Can you work these out from the model? Positions are in its coordinate system, mm. Face numbers are marked on the shaded views. A direction names the side the tool comes from. Coordinates: 2 decimals unless noted, no trailing zeros. Order: outer loops, then holes, each group sorted by start corner. A loop starts at its lowest first (then second) coordinate and runs counter-clockwise, first axis right, second up. Notation, with made-up numbers: (62.5, 70) -> (91.5, 70) arc R33 ccw to (91.5, 99) -> close; hole circle Ø9 at (51.25, -39). An arc over 180 degrees is marked (long way). Write item = value, one per line.
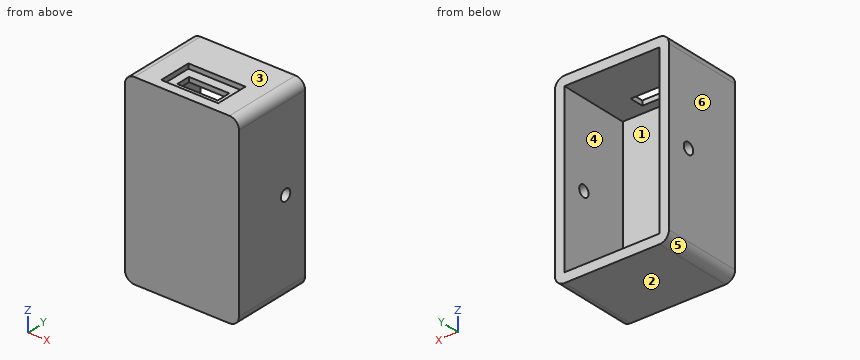
```python
from build123d import *

# Parameters (mm, degrees)
IZIM1_W                     = 24
IZIM1_H                     = 39
Y_KSEKLIK_EKSTR_ZYON1_DEPTH = 17
RADYUS1_R                   = 2
BO_ALTMA1_START             = -12.470588235
BO_ALTMA1_OUTLINE_W         = 15
BO_ALTMA1_OUTLINE_H         = 35
BO_ALTMA1_DEPTH             = 20
IZIM2_W                     = 8.5
IZIM2_H                     = 3
KES_EKSTR_ZYON1_DEPTH       = 17
IZIM3_W                     = 12
IZIM3_H                     = 7
KES_EKSTR_ZYON2_DEPTH       = 1
IZIM5_R                     = 1.2
KES_EKSTR_ZYON3_DEPTH       = 30


# Read off the part's stored shape, not the designer's step: İç Boşaltma1
with BuildPart() as part:
    # Çizim1 → Yükseklik-Ekstrüzyon1 (new body)
    with BuildSketch(Plane(origin=(0, 0, 0), x_dir=(1, 0, 0), z_dir=(0, 1, 0))):
        with Locations((-2.470588235, -5.382352941)):
            Rectangle(IZIM1_W, IZIM1_H)
    extrude(amount=Y_KSEKLIK_EKSTR_ZYON1_DEPTH)

    # Radyus1
    radyus1_edges = [part.edges().sort_by_distance(p)[0] for p in [
        (-14.470588235, 8.5, -14.117647059),
        (9.529411765, 8.5, -14.117647059),
        (9.529411765, 8.5, 24.882352941),
        (-14.470588235, 8.5, 24.882352941),
    ]]
    fillet(radyus1_edges, radius=RADYUS1_R)

    # İç Boşaltma1 outline → İç Boşaltma1 (cut)
    with BuildSketch(Plane.YZ.offset(BO_ALTMA1_START)):
        with Locations((9.5, 5.382352941)):
            Rectangle(BO_ALTMA1_OUTLINE_W, BO_ALTMA1_OUTLINE_H)
    extrude(amount=BO_ALTMA1_DEPTH, mode=Mode.SUBTRACT)

    # Çizim2 → Kes-Ekstrüzyon1 (cut)
    with BuildSketch(Plane.XY.offset(24.882352941)):
        with Locations((-2.470588235, 5.5)):
            Rectangle(IZIM2_W, IZIM2_H)
    extrude(amount=-KES_EKSTR_ZYON1_DEPTH, mode=Mode.SUBTRACT)

    # Çizim3 → Kes-Ekstrüzyon2 (cut)
    with BuildSketch(Plane.XY.offset(24.882352941)):
        with Locations((-2.470588235, 5.5)):
            Rectangle(IZIM3_W, IZIM3_H)
    extrude(amount=-KES_EKSTR_ZYON2_DEPTH, mode=Mode.SUBTRACT)

    # Çizim5 → Kes-Ekstrüzyon3 (cut)
    with BuildSketch(Plane(origin=(9.529411765, 0, 0), x_dir=(0, 0, -1), z_dir=(1, 0, 0))):
        with Locations((-5.382352941, 12)):
            Circle(IZIM5_R)
    extrude(amount=-KES_EKSTR_ZYON3_DEPTH, mode=Mode.SUBTRACT)


solid = part.part
```
Item 1: For the marked faces 1 and 2, which set-ups out of +Z, -Z, +X, -X, +Y, -Y let a thin tool reach every point of the face, with its end or its side?
A:
face_1 = +Y
face_2 = -Z, +X, -X, +Y, -Y
Item 2: I want a section at D-D, the plane z = -3.5. Please give me the cut outline in (x, y).
A:
outline = (-14.47, 0) -> (9.53, 0) -> (9.53, 17) -> (7.53, 17) -> (7.53, 2) -> (-12.47, 2) -> (-12.47, 17) -> (-14.47, 17) -> close
Item 3: I want a section at C-C, the plane y = 14. Please give me the cut outline in (x, z), plus the area to 3 significant figures.
A:
outline = (-14.47, -12.12) arc R2 ccw to (-12.47, -14.12) -> (7.53, -14.12) arc R2 ccw to (9.53, -12.12) -> (9.53, 22.88) arc R2 ccw to (7.53, 24.88) -> (-12.47, 24.88) arc R2 ccw to (-14.47, 22.88) -> close; hole (-12.47, -12.12) -> (7.53, -12.12) -> (7.53, 22.88) -> (-12.47, 22.88) -> close
area = 233 mm2
Item 4: I'm going to push flat-ended pins straight in: P1, Ø2, axis at x = -0.5, y = 7.5, coming from the +Z side; P2, Ø0.8, axis at x = -1, z = 23.5, coming from the -Y side; P3, Ø1.1, axis at y = 5.5, z = 24, coming from the -X side; P4, Ø1.4, axis at y = 12, z = 5.38, coming from the +X side. Where does each tip first touch, or does it pass through?
A:
P1 = 23.88
P2 = 0
P3 = -14.39
P4 = through
Item 5: If we mould it in two halves opening along Z, with no side actions, what happens to the marked faces 3, 4, 5 and 6? For each: pulls with the +Z half, pulls with the -Z half, needs draft (parallel to the pull), parting line crosses it, or undercut.
A:
face_3 = pulls with the +Z half
face_4 = undercut
face_5 = pulls with the -Z half
face_6 = needs draft
Item 6: I want a section at B-B, the plane y = 12. Please give me the cut outline in (x, z).
A:
outline = (-14.47, -12.12) arc R2 ccw to (-12.47, -14.12) -> (7.53, -14.12) arc R2 ccw to (9.53, -12.12) -> (9.53, 4.18) -> (7.53, 4.18) -> (7.53, -12.12) -> (-12.47, -12.12) -> (-12.47, 4.18) -> (-14.47, 4.18) -> close; (-14.47, 6.58) -> (-12.47, 6.58) -> (-12.47, 22.88) -> (7.53, 22.88) -> (7.53, 6.58) -> (9.53, 6.58) -> (9.53, 22.88) arc R2 ccw to (7.53, 24.88) -> (-12.47, 24.88) arc R2 ccw to (-14.47, 22.88) -> close
Item 7: I want a section at A-A, the plane x = 0.75. Please give me the cut outline in (y, z).
A:
outline = (0, -14.12) -> (17, -14.12) -> (17, -12.12) -> (2, -12.12) -> (2, 22.88) -> (4, 22.88) -> (4, 23.88) -> (2, 23.88) -> (2, 24.88) -> (0, 24.88) -> close; (7, 22.88) -> (17, 22.88) -> (17, 24.88) -> (9, 24.88) -> (9, 23.88) -> (7, 23.88) -> close
Item 8: If I drill on probe 1 along X at (y, z) = (3.5, -7); probe 2 along Z at (x, y) = (6.5, 4.25); probe 3 along Y at (x, z) = (-5, 1), over which ranges is the centre line in solid material (lowest first)?
A:
probe_1 = -14.47 to -12.47, 7.53 to 9.53
probe_2 = -14.12 to -12.12, 22.88 to 24.88
probe_3 = 0 to 2
